The listing builds one solid part. Answer for the finished solid, in the listing's coordinates (mm). Face numbers are marked on the shaded views. Coordinates: 2 decimals unless noted, no trailing zeros. Loops run counter-clockwise (first coordinate to the right, second up) from the corner with the lowest first, then second, coordinate; pieces in that order, holes last. Notation, with made-up numbers: M 59,-9.75 L 93,-9.75 A33 cw 93,25.25 Z; hole C -24,20 d5. An arc over 180 degrees is marked long. Answer in a Markdown table with one row per item. Add a question column.
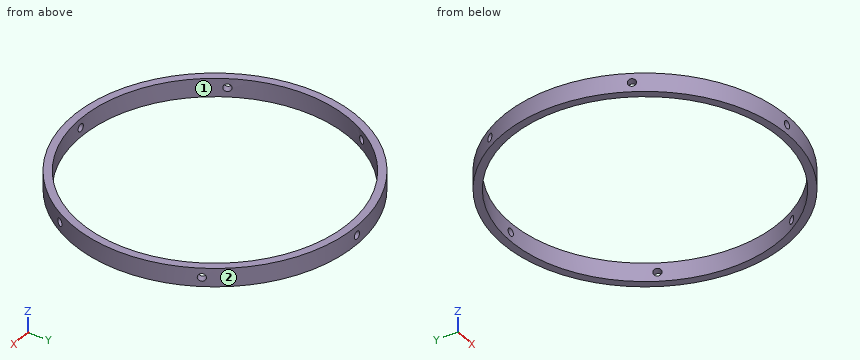
Autodesk Inventor part; units mm, degrees
ref_plane "Work Plane1" through (0, 92.5, 0) normal (0, 1, 0) x (-1, 0, 0)
ref_plane "YZ Plane" through (0, 0, 0) normal (1, 0, 0) x (0, 1, 0)
ref_plane "XY Plane" through (0, 0, 0) normal (0, 0, 1) x (1, 0, 0)
sketch "Sketch1" plane through (0, 0, 0) normal (0, 0, 1) x (1, 0, 0)
  circle A0 centre (0, 0) radius 92.5
  circle A1 centre (0, 0) radius 87.5
  dimension "d0" = 185
  dimension "d1" = 175
extrude "Extrusion1" add sketch "Sketch1" along normal mid plane 12
ref_plane "Work Plane1" through (0, 92.5, 0) normal (0, 1, 0) x (-1, 0, 0)
sketch "Sketch2" plane through (0, 92.5, 0) normal (0, 1, 0) x (-1, 0, 0)
  point P0 (0, 0)
  point P1 (0, 0)
hole "Hole1" at (0, 92.5, 0) direction (0, -1, 0) diameter 5 depth 6
pattern_circular "Circular Pattern1" count 6 over 360 about axis through (0, 0, 0) along (0, 0, 1) of "Hole1"
properties part number "22.3" material "Lead"
(1) Straight lines are drawn through the part: line 1 (Z direction, x = 0, y = 91.15); line 2 (X direction, y = -69, z = -3.75); line 3 (Y direction, x = 0, z = 3.25). For each, find the intervals that lie inside material, in ascending order.
(2) A cutting plane is placed at B-B (z = 0). Give the vertices of the cut face in (x, y), plus the area to 3 significant figures.
(3) A cutting plane is placed at D-D (x = 70). Give the vertices of the cut face in (y, z).
(4) The mould has two halves that part along X. Classify the marked faces 1 and 2: released by +X, released by -X, zero draft, split by the parting line, or undercut.
(5) Each of these flat-tipped pins is pushed along its axis until it touches: pin 1 (3 mm diameter, centred on x = -29, z = 0, fed in from -Y); pin 2 (6 mm diameter, centred on x = 18, z = 1, fed in from -Y); pin 3 (1.5 mm diameter, centred on y = -44.5, z = 5, fed in from -X). Where does it stop, or does it pass through?
(6) A cutting plane is placed at A-A (y = 0). Give the vertices of the cut face in (x, z).
(7) A cutting plane is placed at C-C (x = 0). Give the vertices of the cut face in (y, z), plus the area to 3 significant figures.
Solved:
| question | item | result |
|---|---|---|
| 1 | line 1 | z = -6 to -2.5, 2.5 to 6 |
| 1 | line 2 | x = -61.61 to -53.81, 53.81 to 61.61 |
| 1 | line 3 | y = -92.5 to -87.5, 87.5 to 92.5 |
| 2 | outline | M -81.33,-44.07 L -77,-41.57 A87.5 cw -77,41.57 L -81.33,44.07 A92.5 ccw Z; M -78.83,-48.4 A92.5 ccw -2.5,-92.47 L -2.5,-87.46 A87.5 cw -74.5,-45.9 Z; M -78.83,48.4 L -74.5,45.9 A87.5 cw -2.5,87.46 L -2.5,92.47 A92.5 ccw Z; M 2.5,-92.47 A92.5 ccw 78.83,-48.4 L 74.5,-45.9 A87.5 cw 2.5,-87.46 Z; M 2.5,87.46 A87.5 cw 74.5,45.9 L 78.83,48.4 A92.5 ccw 2.5,92.47 Z; M 77,-41.57 L 81.33,-44.07 A92.5 ccw 81.33,44.07 L 77,41.57 A87.5 cw Z |
| 2 | area | 2,680 mm² |
| 3 | outline | M -60.47,-6 L -52.5,-6 L -52.5,6 L -60.47,6 Z; M 52.5,-6 L 60.47,-6 L 60.47,6 L 52.5,6 Z |
| 4 | face 1 | undercut |
| 4 | face 2 | split by the parting line |
| 5 | pin 1 | stops at y = -88.32 |
| 5 | pin 2 | stops at y = -91.28 |
| 5 | pin 3 | stops at x = -81.5 |
| 6 | outline | M -92.5,-6 L -87.5,-6 L -87.5,6 L -92.5,6 Z; M 87.5,-6 L 92.5,-6 L 92.5,6 L 87.5,6 Z |
| 7 | outline | M -92.5,-6 L -87.5,-6 L -87.5,-2.5 L -92.5,-2.5 Z; M -92.5,2.5 L -87.5,2.5 L -87.5,6 L -92.5,6 Z; M 87.5,-6 L 92.5,-6 L 92.5,-2.5 L 87.5,-2.5 Z; M 87.5,2.5 L 92.5,2.5 L 92.5,6 L 87.5,6 Z |
| 7 | area | 70.0 mm² |
